The listing builds one solid part. Answer for the finished solid, in the listing's coordinates (mm). Face numbers are marked on the shaded views. A direction names the side the tool comes from. Give positions to 0.01 mm unless a question says otherwise; leave off trailing zeros. Order: outer loops, then holes, each group sorted by start corner. A loop starts at its lowest first (then second) coordinate and runs counter-clockwise, first axis right, second up. Notation, with made-up numbers: (-3, -26) - (33, -26) arc R27 cw to (33, -3) - close; hole circle Ø7 at (-7.75, -6.5). An arc over 180 degrees is marked (long way). Answer in a Markdown table with one row per item.
Autodesk Fusion 360 part; units mm, degrees
sketch "Plate" plane through (0, 0, 0) normal (0, 1, 0) x (1, 0, 0)
  line L0 (0, 0) -> (11, 0)
  line L1 (11, 0) -> (11, -20)
  line L2 (11, -20) -> (0, -20)
  line L3 (0, -20) -> (0, 0)
  dimension "d174" = 11
  dimension "d175" = 20
extrude "Plate (1)" add sketch "Plate" along normal mid plane 33 from surface at 4.5
sketch "Screw hole" plane through (0, 0, 0) normal (0, 1, 0) x (1, 0, 0)
  line L0 (-1, -7.6) -> (12, -7.6)
  line L1 (12, -7.6) -> (12, -12.4)
  line L2 (12, -12.4) -> (-1, -12.4)
  line L3 (-1, -12.4) -> (-1, -7.6)
  dimension "d179" = 12
  dimension "d180" = 7.6
  dimension "d181" = 13
  dimension "d182" = 4.8
extrude "Screw hole (1)" cut sketch "Screw hole" along normal mid plane 16.8 from surface at 7.52
sketch "Nut cavity" plane through (0, 0, 0) normal (0, 1, 0) x (1, 0, 0)
  line L0 (3.6, -6.3) -> (7, -6.3)
  line L1 (7, -6.3) -> (7, -13.7)
  line L2 (7, -13.7) -> (3.6, -13.7)
  line L3 (3.6, -13.7) -> (3.6, -6.3)
  dimension "d186" = 7
  dimension "d187" = 6.3
  dimension "d188" = 3.4
  dimension "d189" = 7.4
extrude "Nut cavity (1)" cut sketch "Nut cavity" along normal mid plane 19.4 from surface at 7.52
sketch "Nut entry" plane through (0, 0, 0) normal (0, 1, 0) x (1, 0, 0)
  line L0 (3.6, -12.7) -> (7, -12.7)
  line L1 (7, -12.7) -> (7, -21)
  line L2 (7, -21) -> (3.6, -21)
  line L3 (3.6, -21) -> (3.6, -12.7)
  dimension "d193" = 7
  dimension "d194" = 12.7
  dimension "d195" = 3.4
  dimension "d196" = 8.3
extrude "Nut entry (1)" cut sketch "Nut entry" along normal mid plane 7.4 from surface at 1.52
sketch "Cavity roof" plane through (0, 0, 0) normal (0, 0, 1) x (1, 0, 0)
  line L0 (3.6, -2.18) -> (7, -2.18)
  line L1 (7, -2.18) -> (5.3, -3.88)
  line L2 (5.3, -3.88) -> (3.6, -2.18)
  dimension "d200" = 3.6
  dimension "d201" = 2.18
  dimension "d202" = 7
  dimension "d203" = 5.3
  dimension "d204" = 1.7
extrude "Cavity roof (1)" cut sketch "Cavity roof" along normal mid plane 15.7 from surface at 13.15
equation "bracketWidth = 24.0 mm"
equation "plateHeight = 20.0 mm"
equation "plateInboardExtension = 9.0 mm"
equation "boardThickness = 6.0 mm"
equation "screwLength = 15.0 mm"
equation "screwDiameter = 4.0 mm"
equation "screwClearance = 0.8 mm"
equation "screwTipClearance = 2.0 mm"
equation "screwSlotWidth = screwDiameter + screwClearance"
equation "nutAcrossFlats = 7.0 mm"
equation "nutThickness = 3.0 mm"
equation "nutChannelClearance = 0.4 mm"
equation "nutChannelHeight = nutAcrossFlats + nutChannelClearance"
equation "plateThickness = screwLength - boardThickness + screwTipClearance"
equation "mountTravel = 12.0 mm"
equation "nutChannelLength = mountTravel + nutAcrossFlats + nutChannelClearance"
equation "screwSlotLength = mountTravel + screwSlotWidth"
equation "topMountZ = 10.0 mm"
equation "mountOffsetY = 7.52 mm"
equation "slotOvershoot = 1.0 mm"
equation "nutCavityClearance = 0.4 mm"
equation "nutWallThickness = 4.0 mm"
equation "nutCavityDepth = nutThickness + nutCavityClearance"
equation "nutRoofDepth = nutCavityDepth / 2"
equation "d174 = plateThickness"
equation "d175 = plateHeight"
equation "d176 = plateInboardExtension / 2"
equation "d177 = bracketWidth + plateInboardExtension"
equation "d179 = plateThickness + slotOvershoot"
equation "d180 = topMountZ - screwSlotWidth / 2"
equation "d181 = plateThickness + 2 * slotOvershoot"
equation "d182 = screwSlotWidth"
equation "d183 = mountOffsetY"
equation "d184 = screwSlotLength"
equation "d186 = plateThickness - nutWallThickness"
equation "d187 = topMountZ - nutChannelHeight / 2"
equation "d188 = nutCavityDepth"
equation "d189 = nutChannelHeight"
equation "d190 = mountOffsetY"
equation "d191 = nutChannelLength"
equation "d193 = plateThickness - nutWallThickness"
equation "d194 = topMountZ + nutChannelHeight / 2 - slotOvershoot"
equation "d195 = nutCavityDepth"
equation "d196 = plateHeight - topMountZ - nutChannelHeight / 2 + 2 * slotOvershoot"
equation "d197 = mountOffsetY - mountTravel / 2"
equation "d198 = nutChannelHeight"
equation "d200 = plateThickness - nutWallThickness - nutCavityDepth"
equation "d201 = -( mountOffsetY - nutChannelLength / 2 )"
equation "d202 = plateThickness - nutWallThickness"
equation "d203 = plateThickness - nutWallThickness - nutCavityDepth / 2"
equation "d204 = nutRoofDepth"
equation "d205 = ( topMountZ - nutChannelHeight / 2 + plateHeight ) / 2"
equation "d206 = plateHeight - topMountZ + nutChannelHeight / 2 + 2 * slotOvershoot"
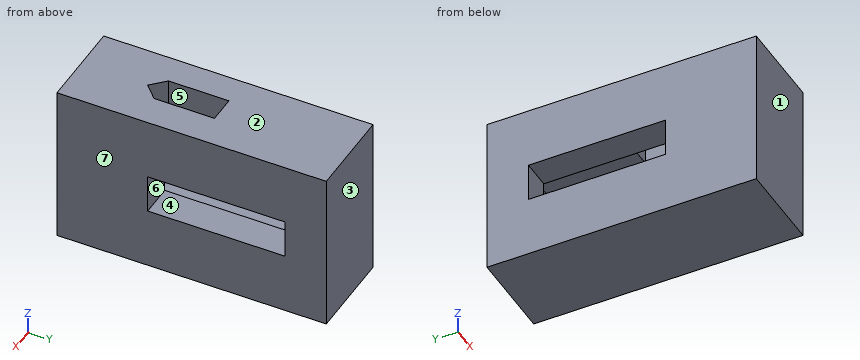
Item 1: Consider line 1 (Z direction, x = 4.5, y = 17); line 2 (Z direction, x = 3.25, y = 2); line 3 (Y direction, x = 7.5, z = 10.75). Determine where each line is inside the solid, lowest interval first.
Answer block:
| item | result |
|---|---|
| line 1 | 0 to 6.3, 13.7 to 20 |
| line 2 | 0 to 7.6, 12.4 to 20 |
| line 3 | -12 to -0.88, 15.92 to 21 |
Item 2: Which of the six approach directions +Z, -Z, +X, -X, +Y, -Y give full straight-line access (tool end or side, diameter ignored) to the marked faces 5, 6 and 7?
Answer block:
| item | result |
|---|---|
| face 5 | none |
| face 6 | +X, -X |
| face 7 | +Z, -Z, +X, +Y, -Y |
Item 3: Find section D-D on x = 2.25. Write down the section's boundary in (y, z), then the cut area to 3 significant figures.
Answer block:
| item | result |
|---|---|
| outline | (-12, 0) - (21, 0) - (21, 20) - (-12, 20) - close; hole (-0.88, 7.6) - (15.92, 7.6) - (15.92, 12.4) - (-0.88, 12.4) - close |
| area | 579 mm² |
Item 4: Find section C-C on y = 0.5. Write down the section's boundary in (x, z).
Answer block:
| item | result |
|---|---|
| outline | (0, 0) - (11, 0) - (11, 7.6) - (7, 7.6) - (7, 6.3) - (3.6, 6.3) - (3.6, 7.6) - (0, 7.6) - close; (0, 12.4) - (3.6, 12.4) - (3.6, 20) - (0, 20) - close; (7, 12.4) - (11, 12.4) - (11, 20) - (7, 20) - close |
Item 5: Determine the mould class of the marked faces 1, 2, 3 and 4 for opening direction Y: pulls with the +Y half, pulls with the -Y half, needs draft (parallel to the pull), parting line crosses it, or undercut.
Answer block:
| item | result |
|---|---|
| face 1 | pulls with the -Y half |
| face 2 | needs draft |
| face 3 | pulls with the +Y half |
| face 4 | undercut |
Item 6: Find section A-A on z = 10. Write down the section's boundary in (x, y), then the cut area to 3 significant figures.
Answer block:
| item | result |
|---|---|
| outline | (0, -12) - (11, -12) - (11, -0.88) - (7, -0.88) - (7, -2.18) - (5.3, -3.88) - (3.6, -2.18) - (3.6, -0.88) - (0, -0.88) - close; (0, 15.92) - (3.6, 15.92) - (3.6, 17.22) - (7, 17.22) - (7, 15.92) - (11, 15.92) - (11, 21) - (0, 21) - close |
| area | 166 mm² |
Item 7: Each of these flat-tipped pins is pushed along its axis until it touches: P1, Ø1, axis at x = 6, y = 4, coming from the +Z side; P2, Ø1.1, axis at x = 1.5, y = 9, coming from the -Z side. Where does it stop, or does it pass through?
Answer block:
| item | result |
|---|---|
| P1 | z = 6.3 |
| P2 | z = 0 |
Item 8: Find section B-B on y = 8. Write down the section's boundary in (x, z), then the cut area to 3 significant figures.
Answer block:
| item | result |
|---|---|
| outline | (0, 0) - (11, 0) - (11, 7.6) - (7, 7.6) - (7, 6.3) - (3.6, 6.3) - (3.6, 7.6) - (0, 7.6) - close; (0, 12.4) - (3.6, 12.4) - (3.6, 13.7) - (7, 13.7) - (7, 12.4) - (11, 12.4) - (11, 20) - (0, 20) - close |
| area | 158 mm² |
